```python
from build123d import *

# Parameters (mm, degrees)
F0_R     = 1
F1_DEPTH = 1
F2_R     = 3


with BuildPart() as f1:
    # F0 (on Top) → F1 (new body)
    with BuildSketch(Plane.XY):
        with BuildLine():
            Line((24, 24), (0, 24))
            Line((0, 24), (-20, 24))
            Line((-20, 24), (-27, 8.8345631957))
            Line((-27, 8.8345631957), (-27, 0))
            Line((-27, 0), (-27, -8.8345631957))
            Line((-27, -8.8345631957), (-20, -24))
            Line((-20, -24), (0, -24))
            Line((0, -24), (24, -24))
            Line((24, -24), (24, -36))
            Line((24, -36), (33, -36))
            ThreePointArc((33, -36), (49.3356561573, 0), (33, 36))
            Line((33, 36), (24, 36))
            Line((24, 36), (24, 24))
        make_face()
        with Locations((-11.5, -22)):
            Circle(F0_R, mode=Mode.SUBTRACT)
        with Locations((11.5, -22)):
            Circle(F0_R, mode=Mode.SUBTRACT)
        with Locations((-11.5, 22)):
            Circle(F0_R, mode=Mode.SUBTRACT)
        with Locations((11.5, 22)):
            Circle(F0_R, mode=Mode.SUBTRACT)
    extrude(amount=F1_DEPTH)

    # F2
    f2_edges = [f1.edges().sort_by_distance(p)[0] for p in [
        (24, -24, 0.5),
        (24, -36, 0.5),
        (24, 24, 0.5),
        (24, 36, 0.5),
    ]]
    fillet(f2_edges, radius=F2_R)


solid = f1.part
```
The listing builds one solid part. Answer for the finished solid, in the listing's coordinates (mm). Coordinates: 2 decimals unless noted, no trailing zeros. Write each loop counter-clockwise with the first axis right and the second up, starting at its lowest first coordinate (ties: lowest second). Pieces come first, ordered by that corner, then holes.
Q1. Find the intervals of material crossed by line 1 along Y through (x, z) = (11.5, 0.55); line 2 along Y through (x, z) = (8, 0.5); line 3 along Y through (x, z) = (23, 0.6), in increasing order.
Returned:
line 1: y = -24 to -23, -21 to 21, 23 to 24
line 2: y = -24 to 24
line 3: y = -24.76 to 24.76
Q2. Section D-D, the plane y = -11 is taken. Write down the section's boundary in (x, z), then the cut area to 3 significant figures.
Returned:
outline: (-26, 0) - (48.05, 0) - (48.05, 1) - (-26, 1) - close
area: 74.1 mm2
Q3. Section A-A, the plane x = 11.5 is taken. Write down the section's boundary in (y, z).
Returned:
outline: (-24, 0) - (-23, 0) - (-23, 1) - (-24, 1) - close; (-21, 0) - (21, 0) - (21, 1) - (-21, 1) - close; (23, 0) - (24, 0) - (24, 1) - (23, 1) - close
Q4. Section C-C, the plane y = -22 is taken. Write down the section's boundary in (x, z).
Returned:
outline: (-20.92, 0) - (-12.5, 0) - (-12.5, 1) - (-20.92, 1) - close; (-10.5, 0) - (10.5, 0) - (10.5, 1) - (-10.5, 1) - close; (12.5, 0) - (43.98, 0) - (43.98, 1) - (12.5, 1) - close
Q5. Section B-B, the plane z = 0.15 is taken. Write down the section's boundary in (x, y), then the cut area to 3 significant figures.
Returned:
outline: (-27, -8.83) - (-20, -24) - (21, -24) arc R3 cw to (24, -27) - (24, -33) arc R3 ccw to (27, -36) - (33, -36) arc R47.84 ccw to (33, 36) - (27, 36) arc R3 ccw to (24, 33) - (24, 27) arc R3 cw to (21, 24) - (-20, 24) - (-27, 8.83) - close; hole circle Ø2 at (-11.5, -22); hole circle Ø2 at (-11.5, 22); hole circle Ø2 at (11.5, -22); hole circle Ø2 at (11.5, 22)
area: 3,790 mm2
Q6. Given P1, Ø2.5, axis at x = 11.5, y = 22, coming from the -Z side; P2, Ø0.5, axis at y = -30, z = 0.5, coming from the -X side; P3, Ø0.5, axis at x = 6.5, z = 0.5, coming from the -Y side, each flat-ended and moving along its own axis, determine where each tip first touches the part or whether it passes through.
Returned:
P1: stops at z = 0
P2: stops at x = 24
P3: stops at y = -24
Q7. The mould has two halves that part along X. Classify faces 1 (the cylindrical face through (-11.717, -22.976, 0.493)), 2 (the flat face through (-23.451, 16.523, 0.493)), 3 (the cylindrical face through (49.332, -0.571, 0.493)): released by +X, released by -X, zero draft, split by the parting line, or undercut.
Returned:
face 1: undercut
face 2: released by -X
face 3: released by +X
